from build123d import *

# Parameters (mm, degrees)
F1_DEPTH = 25.4


with BuildPart() as f1:
    # F0 (on Front) → F1 (new body)
    with BuildSketch(Plane.XZ):
        Polygon((10.893908, 33.528), (0, 33.528), (-10.893908, 33.528), (-28.52062, 20.721444), (-35.253425, 0), (-28.52062, -20.721444), (-10.893908, -33.528), (10.893908, -33.528), (28.52062, -20.721444), (35.253425, 0), (28.52062, 20.721444), align=None)
        Polygon((-5.446954, 16.764), (0, 16.764), (5.446954, 16.764), (14.26031, 10.360722), (17.626713, 0), (14.26031, -10.360722), (5.446954, -16.764), (-5.446954, -16.764), (-14.26031, -10.360722), (-17.626713, 0), (-14.26031, 10.360722), align=None, mode=Mode.SUBTRACT)
    extrude(amount=F1_DEPTH)


solid = f1.part
The model under review builds one solid part; all positions refer to its coordinate system, in mm. A direction names the side the tool comes from. Give positions to 0.01 mm unless a question says otherwise; leave off trailing zeros. Order: outer loops, then holes, each group sorted by start corner. A loop starts at its lowest first (then second) coordinate and runs counter-clockwise, first axis right, second up. Notation, with made-up numbers: M 8,-16 L 56,-16 A7 ccw 56,-10 Z; hole C -24.75,78 d10. An arc over 180 degrees is marked long. Use one line per item in the form item = value. Start each with the question number.
Item 1: We need section B-B on y = -23.25. Give the boundary of the cut face in (x, z), plus the area to 3 significant figures.
Item 2: To check wall thickness, follow line 1 along Z through (x, y) = (0.5, -14.25); line 2 along Z through (x, y) = (7, -11); line 3 along X through (y, z) = (-22.75, -16). State the ranges of each line that lie inside material, in increasing order. Write a range as from..to.
Item 3: For faces 1 (the flat face through (-19.584, -12.522, 27.214)), 2 (the flat face through (0, -13, 16.764)), list the 3-axis set-ups (+Z, -Z, +X, -X, +Y, -Y) from which the entire face can be reached by the end or side of a thin tool; tool diameter is ignored.
Item 4: Insertion check: pin 1 Ø8 at (y, z) = (-17, 22) entering from -X; pin 2 Ø10 at (y, z) = (-14, -24.5) entering from +X; pin 3 Ø10 at (y, z) = (-5.5, -11.5) entering from -X. Each pin has a flat end and moves straight along its axis. Give the tip position at first contact, or say it passes through.
Item 5: We need section A-A on x = 16. Give the boundary of the cut face in (y, z).
Item 6: The part is to be moulded in two halves that separate along X. For faces 3 (the flat face through (19.831, -12.522, 27.035)), 4 (the flat face through (-9.915, -12.522, 13.518)), 5 (the flat face through (-19.831, -12.522, -27.035)), say which applies: pulls with the +X half, pulls with the -X half, needs draft (parallel to the pull), parting line crosses it, or undercut.
Item 7: We need section C-C on z = 12. Give the boundary of the cut face in (x, y), plus the area to 3 significant figures.
Item 8: We need section D-D on z = 24. Give the boundary of the cut face in (x, y), plus the area to 3 significant figures.
Completed:
q1.outline = M -35.25,0 L -28.52,-20.72 L -10.89,-33.53 L 10.89,-33.53 L 28.52,-20.72 L 35.25,0 L 28.52,20.72 L 10.89,33.53 L -10.89,33.53 L -28.52,20.72 Z; hole M -17.63,0 L -14.26,-10.36 L -5.45,-16.76 L 5.45,-16.76 L 14.26,-10.36 L 17.63,0 L 14.26,10.36 L 5.45,16.76 L -5.45,16.76 L -14.26,10.36 Z
q1.area = 2,740 mm²
q2.line_1 = -33.53..-16.76, 16.76..33.53
q2.line_2 = -33.53..-15.64, 15.64..33.53
q2.line_3 = -30.05..-6.5, 6.5..30.05
q3.face_1 = +Z, -X, +Y, -Y
q3.face_2 = +Y, -Y
q4.pin_1 = -29.4
q4.pin_2 = 28.92
q4.pin_3 = -33.14
q5.outline = M -25.4,-29.82 L 0,-29.82 L 0,-5.01 L -25.4,-5.01 Z; M -25.4,5.01 L 0,5.01 L 0,29.82 L -25.4,29.82 Z
q6.face_3 = pulls with the +X half
q6.face_4 = undercut
q6.face_5 = pulls with the -X half
q7.outline = M -31.35,-25.4 L -12,-25.4 L -12,0 L -31.35,0 Z; M 12,-25.4 L 31.35,-25.4 L 31.35,0 L 12,0 Z
q7.area = 983 mm²
q8.outline = M -24.01,-25.4 L 24.01,-25.4 L 24.01,0 L -24.01,0 Z
q8.area = 1,220 mm²
